from build123d import *

# Parameters (mm, degrees)
SKETCH_1_W                  = 85
SKETCH_1_H                  = 36
EXTRUDE_1_DEPTH             = 1.5
SKETCH_2_W                  = 69.2
SKETCH_2_H                  = 29.2
EXTRUDE_2_DEPTH             = 9
CUT_EXTRUDE_1_REACH         = 49.024
SKETCH_3_R                  = 1.35
SKETCH_4_W                  = 62
SKETCH_4_H                  = 19
CUT_EXTRUDE_2_DEPTH         = 0.5
FILLET_1_R                  = 1
CUT_EXTRUDE_3_REACH         = 49.024
SKETCH_5_R                  = 0.4
PATTERN_LINEAR_1_COUNT      = 8
PATTERN_LINEAR_1_PITCH      = 2.54
PATTERN_LINEAR_1_COUNT_DIR2 = 2
PATTERN_LINEAR_1_PITCH_DIR2 = 2.54


with BuildPart() as part:
    # Эскиз1 → Бобышка-Вытянуть1 (new body)
    with BuildSketch(Plane(origin=(0, 0, 0), x_dir=(1, 0, 0), z_dir=(0, 1, 0))):
        Rectangle(SKETCH_1_W, SKETCH_1_H)
    extrude(amount=EXTRUDE_1_DEPTH)

    # Эскиз2 → Бобышка-Вытянуть2 (add)
    with BuildSketch(Plane(origin=(0, 1.5, 0), x_dir=(1, 0, 0), z_dir=(0, 1, 0))):
        Rectangle(SKETCH_2_W, SKETCH_2_H)
    extrude(amount=EXTRUDE_2_DEPTH)

    # Эскиз3 → Вырез-Вытянуть1 (cut, up to next)
    with BuildSketch(Plane(origin=(0, 1.5, 0), x_dir=(1, 0, 0), z_dir=(0, 1, 0)), mode=Mode.PRIVATE) as cut_extrude_1_sk1:
        with Locations(Location((-40, 15.5, 0), (0, 0, 270))):
            Circle(SKETCH_3_R)
    cut_extrude_1_tool1 = extrude(cut_extrude_1_sk1.sketch, amount=-CUT_EXTRUDE_1_REACH, mode=Mode.PRIVATE) & part.part
    # Эскиз3 → Вырез-Вытянуть1 (cut, up to next)
    with BuildSketch(Plane(origin=(0, 1.5, 0), x_dir=(1, 0, 0), z_dir=(0, 1, 0)), mode=Mode.PRIVATE) as cut_extrude_1_sk2:
        with Locations(Location((-40, -15.5, 0), (0, 0, 90))):
            Circle(SKETCH_3_R)
    cut_extrude_1_tool2 = extrude(cut_extrude_1_sk2.sketch, amount=-CUT_EXTRUDE_1_REACH, mode=Mode.PRIVATE) & part.part
    # Эскиз3 → Вырез-Вытянуть1 (cut, up to next)
    with BuildSketch(Plane(origin=(0, 1.5, 0), x_dir=(1, 0, 0), z_dir=(0, 1, 0)), mode=Mode.PRIVATE) as cut_extrude_1_sk3:
        with Locations(Location((40, -15.5, 0), (0, 0, 270))):
            Circle(SKETCH_3_R)
    cut_extrude_1_tool3 = extrude(cut_extrude_1_sk3.sketch, amount=-CUT_EXTRUDE_1_REACH, mode=Mode.PRIVATE) & part.part
    # Эскиз3 → Вырез-Вытянуть1 (cut, up to next)
    with BuildSketch(Plane(origin=(0, 1.5, 0), x_dir=(1, 0, 0), z_dir=(0, 1, 0)), mode=Mode.PRIVATE) as cut_extrude_1_sk4:
        with Locations(Location((40, 15.5, 0), (0, 0, 90))):
            Circle(SKETCH_3_R)
    cut_extrude_1_tool4 = extrude(cut_extrude_1_sk4.sketch, amount=-CUT_EXTRUDE_1_REACH, mode=Mode.PRIVATE) & part.part
    add(cut_extrude_1_tool1.solids().sort_by_distance((-40, 1.5, -15.5))[0], mode=Mode.SUBTRACT)
    add(cut_extrude_1_tool2.solids().sort_by_distance((-40, 1.5, 15.5))[0], mode=Mode.SUBTRACT)
    add(cut_extrude_1_tool3.solids().sort_by_distance((40, 1.5, 15.5))[0], mode=Mode.SUBTRACT)
    add(cut_extrude_1_tool4.solids().sort_by_distance((40, 1.5, -15.5))[0], mode=Mode.SUBTRACT)

    # Эскиз4 → Вырез-Вытянуть2 (cut)
    with BuildSketch(Plane(origin=(0, 10.5, 0), x_dir=(1, 0, 0), z_dir=(0, 1, 0))):
        Rectangle(SKETCH_4_W, SKETCH_4_H)
    extrude(amount=-CUT_EXTRUDE_2_DEPTH, mode=Mode.SUBTRACT)

    # Скругление1
    fillet_1_edges = [part.edges().sort_by_distance(p)[0] for p in [
        (34.6, 10.5, 0),
        (0, 10.5, -14.6),
        (-34.6, 10.5, 0),
        (0, 10.5, 14.6),
    ]]
    fillet(fillet_1_edges, radius=FILLET_1_R)

    # Эскиз5 → Вырез-Вытянуть3 (cut, up to next)
    with BuildSketch(Plane(origin=(0, 1.5, 0), x_dir=(1, 0, 0), z_dir=(0, 1, 0)), mode=Mode.PRIVATE) as cut_extrude_3_sk1:
        with Locations(Location((-40, 8.89, 0), (0, 0, 270))):
            Circle(SKETCH_5_R)
    cut_extrude_3_tool1 = extrude(cut_extrude_3_sk1.sketch, amount=-CUT_EXTRUDE_3_REACH, mode=Mode.PRIVATE) & part.part
    cut_extrude_3 = cut_extrude_3_tool1.solids().sort_by_distance((-40, 1.5, -8.89))[0]
    add(cut_extrude_3, mode=Mode.SUBTRACT)

    # Линейный массив1: Cut-Extrude 3 8 × 2
    with Locations(*[(j * PATTERN_LINEAR_1_PITCH_DIR2, 0, i * PATTERN_LINEAR_1_PITCH) for i in range(PATTERN_LINEAR_1_COUNT) for j in range(PATTERN_LINEAR_1_COUNT_DIR2) if (i, j) != (0, 0)]):
        add(cut_extrude_3, mode=Mode.SUBTRACT)


solid = part.part
CAD build for the part. Positions are in the model's coordinates, mm. A direction names the side the tool comes from. Round coordinates to 2 decimals unless told otherwise and drop trailing zeros. Write each loop counter-clockwise with the first axis right and the second up, starting at its lowest first coordinate (ties: lowest second). Pieces come first, ordered by that corner, then holes. Notation, with made-up numbers: (15, 67.25) -> (50, 67.25) arc R30 cw to (50, 105.25) -> close; hole circle Ø1 at (23, 77.25). An arc over 180 degrees is marked (long way). Answer as a JSON object with one key per item and string values.
(1) Band-saw the part on B-B, the plane x = 40. List the corners of the cut face in (y, z).
Reported:
{"outline": "(0, -18) -> (1.5, -18) -> (1.5, -16.85) -> (0, -16.85) -> close; (0, -14.15) -> (1.5, -14.15) -> (1.5, 14.15) -> (0, 14.15) -> close; (0, 16.85) -> (1.5, 16.85) -> (1.5, 18) -> (0, 18) -> close"}
(2) Pin check, flat tips, straight feed: P1, Ø5, axis at x = 29, z = -5.5, coming from the +Y side; P2, Ø1, axis at x = 14.5, y = 4, coming from the -Z side; P3, Ø6, axis at x = 8, y = 6.5, coming from the +Z side; P4, Ø5.5, axis at x = 8.5, z = -4.5, coming from the +Y side. Stop position of each tip, or through.
Reported:
{"P1": "stops at y = 10.5", "P2": "stops at z = -14.6", "P3": "stops at z = 14.6", "P4": "stops at y = 10"}
(3) Which spindle directions (+Z, -Z, +X, -X, +Y, -Y) get a long thin tool onto all of the face, cutting with end or side? Do faces 5 (the face through (0, 10, 0)), 6 (the face through (34.6, 5, 0)), 7 (the face through (-34.6, 5, 0)), 8 (the face through (0, 5, 14.6)), 9 (the face through (0, 10.5, -10)). Say none if no direction does.
Reported:
{"face 5": "+Y", "face 6": "+Z, -Z, +X, +Y", "face 7": "+Z, -Z, -X, +Y", "face 8": "+Z, +X, -X, +Y", "face 9": "+Z, -Z, +X, -X, +Y"}
(4) Two-plate mould, pull along X, no slides. Class faces 1 (the face through (41.32, 0.76, -15.21)), 2 (the face through (38.68, 0.76, 15.21)), 3 (the face through (42.5, 1, 0)), 4 (the face through (0, 5, -14.6)): +X half, -X half, draft (parallel to the pull), parting line (faces both ways), or undercut.
Reported:
{"face 1": "undercut", "face 2": "undercut", "face 3": "+X half", "face 4": "draft"}
(5) Band-saw the part on A-A, the plane z = 15.5. List the corners of the cut face in (x, y), then the cut area to 3 significant figures.
Reported:
{"outline": "(-42.5, 0) -> (-41.35, 0) -> (-41.35, 1.5) -> (-42.5, 1.5) -> close; (-38.65, 0) -> (38.65, 0) -> (38.65, 1.5) -> (-38.65, 1.5) -> close; (41.35, 0) -> (42.5, 0) -> (42.5, 1.5) -> (41.35, 1.5) -> close", "area": "119 mm^2"}
(6) Band-saw the part on D-D, the plane y = 4.5. List the corners of the cut face in (x, z), then the cut area to 3 significant figures.
Reported:
{"outline": "(-34.6, -14.6) -> (34.6, -14.6) -> (34.6, 14.6) -> (-34.6, 14.6) -> close", "area": "2,020 mm^2"}
(7) Probe probe 1 along X at (y, z) = (0.95, 6.35); probe 2 along Y at (x, z) = (29, 3); probe 3 along X at (y, z) = (5.75, -6.5). List the from-to ranges inside material, lowest first. Write a range as [from, to].
Reported:
{"probe 1": "x = [-42.5, -40.4], [-39.6, -37.86], [-37.06, 42.5]", "probe 2": "y = [0, 10]", "probe 3": "x = [-34.6, 34.6]"}
(8) Band-saw the part on C-C, the plane x = -26. List the corners of the cut face in (y, z), then the cut area to 3 significant figures.
Reported:
{"outline": "(0, -18) -> (1.5, -18) -> (1.5, -14.6) -> (9.5, -14.6) arc R1 ccw to (10.5, -13.6) -> (10.5, -9.5) -> (10, -9.5) -> (10, 9.5) -> (10.5, 9.5) -> (10.5, 13.6) arc R1 ccw to (9.5, 14.6) -> (1.5, 14.6) -> (1.5, 18) -> (0, 18) -> close", "area": "307 mm^2"}
